Read the model definition and answer for the solid it produces. Units are mm, in the model's axes. A direction names the side the tool comes from. Give positions to 0.01 mm unless a question says otherwise; leave off trailing zeros. Write each loop counter-clockwise with the first axis right and the second up, starting at its lowest first coordinate (ties: lowest second). Pieces come first, ordered by that corner, then holes.
```python
from build123d import *

# Parameters (mm, degrees)
SKETCH1_R           = 36.3
SKETCH1_R_2         = 15.5
BOSS_EXTRUDE1_DEPTH = 4


with BuildPart() as part:
    # Sketch1 → Boss-Extrude1 (new body)
    with BuildSketch(Plane(origin=(0, 0, 0), x_dir=(1, 0, 0), z_dir=(0, 1, 0))):
        with Locations(Location((0, 0, 0), (0, 0, 270))):
            Circle(SKETCH1_R)
        with Locations(Location((0, 0, 0), (0, 0, 270))):
            Circle(SKETCH1_R_2, mode=Mode.SUBTRACT)
        Polygon((25.190598923, -4), (22.881197846, 0), (25.190598923, 4), (29.809401077, 4), (32.118802154, 0), (29.809401077, -4), align=None, mode=Mode.SUBTRACT)
        Polygon((-22.881197846, 0), (-25.190598923, 4), (-29.809401077, 4), (-32.118802154, 0), (-29.809401077, -4), (-25.190598923, -4), align=None, mode=Mode.SUBTRACT)
    extrude(amount=BOSS_EXTRUDE1_DEPTH)


solid = part.part
```
Item 1: Find the intervals of material crossed by line 1 along X through (y, z) = (1.8, 0); line 2 along X through (y, z) = (1.35, 6.5); line 3 along X through (y, z) = (1.6, 13), in increasing order.
Result set:
line 1: x = -36.3 to -32.12, -22.88 to -15.5, 15.5 to 22.88, 32.12 to 36.3
line 2: x = -35.71 to -14.07, 14.07 to 35.71
line 3: x = -33.89 to -8.44, 8.44 to 33.89
Item 2: Section D-D (z = -16.5) is taken. Write down the section's boundary in (x, y).
Result set:
outline: (-32.33, 0) - (32.33, 0) - (32.33, 4) - (-32.33, 4) - close
Item 3: This flat-tipped pin is pushed along its axis until it touches: pin 1 Ø1.2 at (x, y) = (26.5, 3) entering from +Z. Where does it stop, or does it pass through?
Result set:
pin 1: stops at z = 25.43
Item 4: Section C-C (z = -5) is taken. Write down the section's boundary in (x, y).
Result set:
outline: (-35.95, 0) - (-14.67, 0) - (-14.67, 4) - (-35.95, 4) - close; (14.67, 0) - (35.95, 0) - (35.95, 4) - (14.67, 4) - close
Item 5: Which of the six approach directions +Z, -Z, +X, -X, +Y, -Y give full straight-line access (tool end or side, diameter ignored) to faces 4 (the flat face through (-27, 2, -4)), 5 (the flat face through (1, 0, 16))?
Result set:
face 4: +Y, -Y
face 5: +Z, -Z, +X, -X, -Y
Item 6: Determine the mould class of faces 1 (the cylindrical face through (-22.088, 1.972, -28.806)), 2 (the flat face through (1, 4, 16)), 3 (the flat face through (-28, 2, 4)) for opening direction Z: pulls with the +Z half, pulls with the -Z half, needs draft (parallel to the pull), parting line crosses it, or undercut.
Result set:
face 1: parting line crosses it
face 2: needs draft
face 3: undercut
Item 7: Section B-B (y = 0.9) is taken. Write down the section's boundary in (x, z), and give its area (3 significant figures).
Result set:
outline: circle Ø72.6 at (0, 0); hole (-32.12, 0) - (-29.81, -4) - (-25.19, -4) - (-22.88, 0) - (-25.19, 4) - (-29.81, 4) - close; hole circle Ø31 at (0, 0); hole (22.88, 0) - (25.19, -4) - (29.81, -4) - (32.12, 0) - (29.81, 4) - (25.19, 4) - close
area: 3,270 mm2
Item 8: Section A-A (x = 0) is taken. Write down the section's boundary in (y, z), and give its area (3 significant figures).
Result set:
outline: (0, -36.3) - (4, -36.3) - (4, -15.5) - (0, -15.5) - close; (0, 15.5) - (4, 15.5) - (4, 36.3) - (0, 36.3) - close
area: 166 mm2
